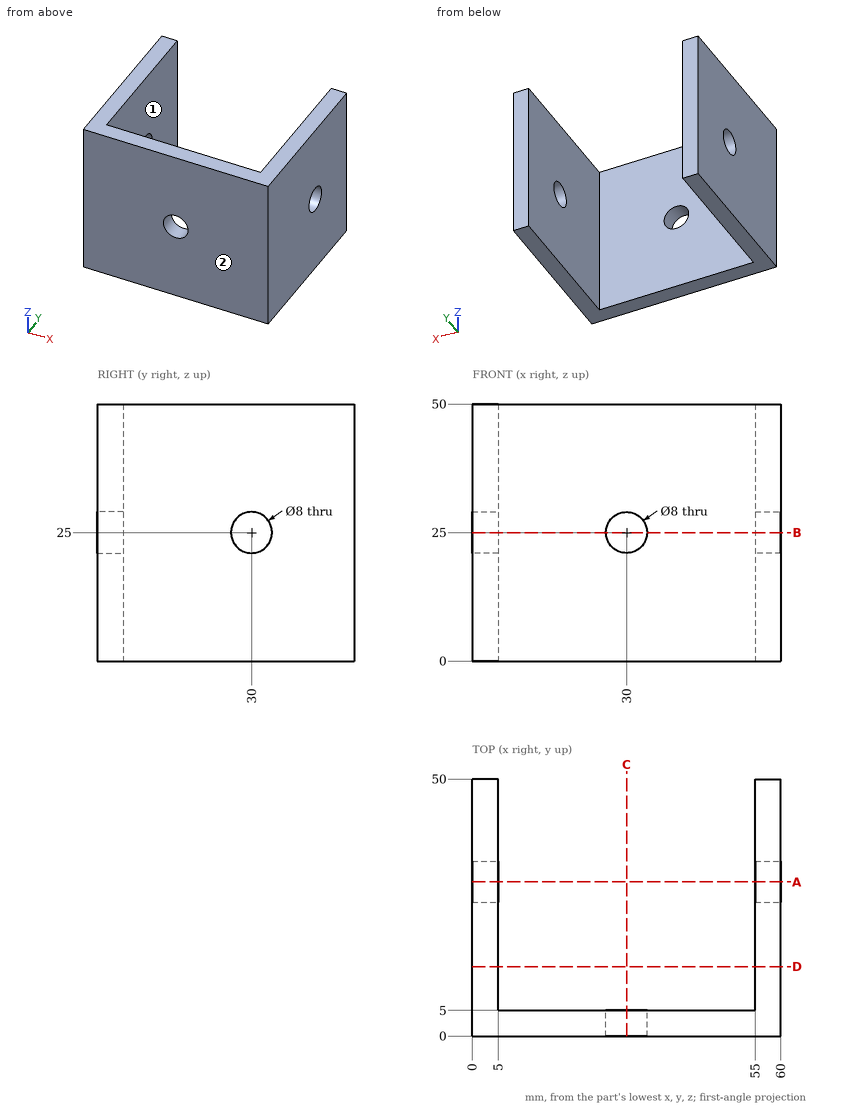
Part print with two shaded views. Sizes in mm from the minimum x, y, z corner. A direction names the side the tool comes from. Round coordinates to 2 decimals unless told otherwise and drop trailing zeros. Loops run counter-clockwise (first coordinate to the right, second up) from the corner with the lowest first, then second, coordinate; pieces in that order, holes last.
1. Slice it at B-B (z = 25). Give the cut face in (x, y).
Solutions:
outline: (0, 0) - (26, 0) - (26, 5) - (5, 5) - (5, 26) - (0, 26) - close; (0, 34) - (5, 34) - (5, 50) - (0, 50) - close; (34, 0) - (60, 0) - (60, 26) - (55, 26) - (55, 5) - (34, 5) - close; (55, 34) - (60, 34) - (60, 50) - (55, 50) - close
2. 3-axis set-ups, long thin cutter, end or side, ignore diameter. For the marked faces 1 and 2: which of +Z, -Z, +X, -X, +Y, -Y reach the whole face in a straight line?
Solutions:
face 1: +Z, -Z, +Y
face 2: +Z, -Z, +X, -X, -Y
3. Slice it at A-A (y = 30). Give the cut face in (x, z), and give its area (3 significant figures).
Solutions:
outline: (0, 0) - (5, 0) - (5, 21) - (0, 21) - close; (0, 29) - (5, 29) - (5, 50) - (0, 50) - close; (55, 0) - (60, 0) - (60, 21) - (55, 21) - close; (55, 29) - (60, 29) - (60, 50) - (55, 50) - close
area: 420 mm2
4. Slice it at D-D (y = 13.5). Give the cut face in (x, z), and give its area (3 significant figures).
Solutions:
outline: (0, 0) - (5, 0) - (5, 50) - (0, 50) - close; (55, 0) - (60, 0) - (60, 50) - (55, 50) - close
area: 500 mm2
5. Drill centre lines: line 1 along X through (y, z) = (1, 25); line 2 along X through (y, z) = (13, 6); line 3 along Y through (x, z) = (50, 29). Where is each one in solid material? Low to high.
Solutions:
line 1: x = 0 to 26, 34 to 60
line 2: x = 0 to 5, 55 to 60
line 3: y = 0 to 5
6. Flat gauge pins, fed straight in: pin 1 (3 mm diameter, centred on x = 47, z = 22, fed in from +Y); pin 2 (7 mm diameter, centred on y = 30, z = 25, fed in from -X). Where does each tip first touch, or does it go through?
Solutions:
pin 1: stops at y = 5
pin 2: passes through
7. Slice it at C-C (x = 30). Give the cut face in (y, z).
Solutions:
outline: (0, 0) - (5, 0) - (5, 21) - (0, 21) - close; (0, 29) - (5, 29) - (5, 50) - (0, 50) - close
